```python
from build123d import *

# Parameters (mm, degrees)
F1_DEPTH  = 1525.228
F3_DEPTH  = 1525.228
F5_D      = 19
F5_DEPTH  = 5
F5_TIP    = 5.7081758808
F7_D      = 9
F7_DEPTH  = 5
F7_TIP    = 2.7038727856
F8_R      = 19.05
F9_DEPTH  = 457.2
F10_R     = 7.5
F11_DEPTH = 120
F12_DEPTH = 20
F16_R     = 7.5
F17_DEPTH = 60
F22_R     = 7.5
F23_DEPTH = 60
F28_D     = 15
F28_DEPTH = 5
F28_TIP   = 4.5064546427
F30_D     = 18
F30_DEPTH = 5
F30_TIP   = 5.4077455712
F32_D     = 10
F32_DEPTH = 5
F32_TIP   = 3.0043030951
F33_W     = 75
F33_H     = 1545.228
F34_DEPTH = 2500


# Not quite as in the source:
# - a feature names something its author has since deleted; it is built from what else it names


with BuildPart() as f1:
    # F0 (on Front) → F1 (new body)
    with BuildSketch(Plane.XZ):
        with BuildLine():
            ThreePointArc((0, 12.7), (3.7197438789, 3.7197438789), (12.7, 0))
            Line((12.7, 0), (63.5, 0))
            ThreePointArc((63.5, 0), (72.4802561211, 3.7197438789), (76.2, 12.7))
            Line((76.2, 12.7), (76.2, 63.5))
            ThreePointArc((76.2, 63.5), (72.4802561211, 72.4802561211), (63.5, 76.2))
            Line((63.5, 76.2), (12.7, 76.2))
            ThreePointArc((12.7, 76.2), (3.7197438789, 72.4802561211), (0, 63.5))
            Line((0, 63.5), (0, 12.7))
        make_face()
    extrude(amount=-F1_DEPTH)

    # F2 (on face) → F3 (cut)
    with BuildSketch(Plane.XZ):
        with BuildLine():
            Line((17.4625, 4.7625), (38.1, 4.7625))
            Line((38.1, 4.7625), (58.7375, 4.7625))
            ThreePointArc((58.7375, 4.7625), (67.7177561211, 8.4822438789), (71.4375, 17.4625))
            Line((71.4375, 17.4625), (71.4375, 58.7375))
            ThreePointArc((71.4375, 58.7375), (67.7177561211, 67.7177561211), (58.7375, 71.4375))
            Line((58.7375, 71.4375), (17.4625, 71.4375))
            ThreePointArc((17.4625, 71.4375), (8.4822438789, 67.7177561211), (4.7625, 58.7375))
            Line((4.7625, 58.7375), (4.7625, 17.4625))
            ThreePointArc((4.7625, 17.4625), (8.4822438789, 8.4822438789), (17.4625, 4.7625))
        make_face()
    extrude(amount=-F3_DEPTH, mode=Mode.SUBTRACT)

    # F5
    with Locations(Plane.YZ.offset(76.2)):
        with Locations((1335.228, 46.2), (1105.028, 46.2), (653.528, 46.2), (381.528, 46.2), (179.528, 46.2)):
            Hole(F5_D / 2, depth=F5_DEPTH)
            with Locations((0, 0, -(F5_DEPTH + F5_TIP / 2))):  # 118° drill point
                Cone(0, F5_D / 2, F5_TIP, mode=Mode.SUBTRACT)

    # F7
    with Locations(Plane.YZ.offset(76.2)):
        with Locations((261.933, 31.2), (501.133, 31.2), (760.333, 31.2), (979.533, 31.2), (1218.698, 31.2)):
            Hole(F7_D / 2, depth=F7_DEPTH)
            with Locations((0, 0, -(F7_DEPTH + F7_TIP / 2))):  # 118° drill point
                Cone(0, F7_D / 2, F7_TIP, mode=Mode.SUBTRACT)

    # F8 (on face) → F9 (join)
    with BuildSketch(Plane.XY.offset(76.2)):
        with Locations((38.1, 30)):
            Circle(F8_R)
    extrude(amount=F9_DEPTH)

    # F10 (on face) → F11 (join)
    with BuildSketch(Plane.XY.offset(76.2)):
        with Locations((20.2, 121.55)):
            Circle(F10_R)
    extrude(amount=F11_DEPTH)

    # F12 (add): a face of the model
    f12_faces = [f1.faces().sort_by_distance(p)[0] for p in [
        (1.0776307345, 1525.228, 38.1),
    ]]
    extrude(f12_faces, amount=F12_DEPTH)

    # F16 (on 3pt) → F17 (join)
    with BuildSketch(Plane.XZ.offset(-129.05)):
        with Locations((0, 76.2)):
            Circle(F16_R)
    extrude(amount=-F17_DEPTH)

    # F22 (on 3pt) → F23 (join)
    with BuildSketch(Plane(origin=(0, 1525.228, 0), x_dir=(-1, 0, 0), z_dir=(0, 1, 0))):
        with Locations((0, 76.2)):
            Circle(F22_R)
    extrude(amount=-F23_DEPTH)

    # F28
    with Locations(Plane.YZ.offset(76.2)):
        with Locations((1442.058, 31.2)):
            Hole(F28_D / 2, depth=F28_DEPTH)
            with Locations((0, 0, -(F28_DEPTH + F28_TIP / 2))):  # 118° drill point
                Cone(0, F28_D / 2, F28_TIP, mode=Mode.SUBTRACT)

    # F30
    with Locations(Plane(origin=(0, 0, 0), x_dir=(0, -1, 0), z_dir=(-1, 0, 0))):
        with Locations((-1385.03, 45.756), (-1244.831, 45.756), (-1104.633, 45.756), (-964.435, 45.756), (-263.443, 45.756), (-179.228, 45.756)):
            Hole(F30_D / 2, depth=F30_DEPTH)
            with Locations((0, 0, -(F30_DEPTH + F30_TIP / 2))):  # 118° drill point
                Cone(0, F30_D / 2, F30_TIP, mode=Mode.SUBTRACT)

    # F32
    with Locations(Plane(origin=(0, 0, 0), x_dir=(0, -1, 0), z_dir=(-1, 0, 0))):
        with Locations((-702.728, 47.406), (-350.228, 47.406)):
            Hole(F32_D / 2, depth=F32_DEPTH)
            with Locations((0, 0, -(F32_DEPTH + F32_TIP / 2))):  # 118° drill point
                Cone(0, F32_D / 2, F32_TIP, mode=Mode.SUBTRACT)

    # F33 (on face) → F34 (cut)
    with BuildSketch(Plane(origin=(0, 0, 0), x_dir=(1, 0, 0), z_dir=(0, 0, -1))):
        with Locations((75.6, -772.614)):
            Rectangle(F33_W, F33_H)
    extrude(amount=-F34_DEPTH, mode=Mode.SUBTRACT)


solid = f1.part
```
Geometry: final body of the model. Coordinates: model frame, mm. A direction names the side the tool comes from. Coordinates: 2 decimals unless noted, no trailing zeros. Loops run counter-clockwise (first coordinate to the right, second up) from the corner with the lowest first, then second, coordinate; pieces in that order, holes last. Notation, with made-up numbers: (67.5, 40) -> (121.5, 40) arc R19 ccw to (121.5, 47) -> close; hole circle Ø1 at (-12.75, 46). An arc over 180 degrees is marked (long way). Use a Markdown table: item, result. Add a question column.
(1) Section query C-C, the plane z = 497. Return loops of the section in (x, y).
(2) Section query B-B, the plane z = 151. Return loops of the section in (x, y), plus the area to 3 significant figures.
(3) Section query D-D, the plane y = 1132. Return loops of the section in (x, z), plus the area to 3 significant figures.
(4) Mould query, pull axis Z, two halves, no side actions, for faces 1 (the flat face through (3, 0, 41)), 2 (the flat face through (4.762, 762, 38)), 3 (the flat face through (25, 762, 0)). Classes: pulls with the +Z half, pulls with the -Z half, needs draft (parallel to the pull), parting line crosses it, or undercut.
(5) Access query for faces 4 (the flat face through (3, 1545.228, 41)), 5 (the cylindrical face through (19.055, 30.419, 301.6)). Directions: +Z, -Z, +X, -X, +Y, -Y. A direction counts if a zero-diameter tool reaches every point of the face in a straight line with its end or side. Return the directions, or none.
(6) Pin query (flat end, axial travel): pin 1 Ø8 at (x, z) = (10, 93.5) entering from -Y; pin 2 Ø7.5 at (x, z) = (-0.5, 77.5) entering from -Y; pin 3 Ø23.5 at (y, z) = (179.228, 45.756) entering from -X; pin 4 Ø16.5 at (x, z) = (3, 76.5) entering from +Y. Return the tip coordinate at first contact, or that it passes through.
(7) Section query A-A, the plane y = 30. Return loops of the section in (x, z).
(8) Line query: line 1 along Z through (x, y) = (15, 145); line 2 along Z through (x, y) = (17, 845); line 3 along X through (y, z) = (879, 33). Output: solid intervals per line, ascending.
Answer:
| question | item | result |
|---|---|---|
| 1 | outline | (38.1, 10.95) -> (38.1, 49.05) arc R19.05 ccw to start |
| 2 | outline | circle Ø15 at (20.2, 121.55); (38.1, 10.95) -> (38.1, 49.05) arc R19.05 ccw to start |
| 2 | area | 747 mm^2 |
| 3 | outline | (0, 12.7) arc R12.7 ccw to (12.7, 0) -> (38.1, 0) -> (38.1, 4.76) -> (17.46, 4.76) arc R12.7 cw to (4.76, 17.46) -> (4.76, 58.74) arc R12.7 cw to (17.46, 71.44) -> (38.1, 71.44) -> (38.1, 76.2) -> (12.7, 76.2) arc R12.7 ccw to (0, 63.5) -> close |
| 3 | area | 680 mm^2 |
| 4 | face 1 | needs draft |
| 4 | face 2 | undercut |
| 4 | face 3 | pulls with the -Z half |
| 5 | face 4 | +Z, -Z, +X, -X, +Y |
| 5 | face 5 | +Z, -X |
| 6 | pin 1 | stops at y = 117.33 |
| 6 | pin 2 | stops at y = 129.05 |
| 6 | pin 3 | stops at x = 0 |
| 6 | pin 4 | stops at y = 1545.23 |
| 7 | outline | (0, 12.7) arc R12.7 ccw to (12.7, 0) -> (38.1, 0) -> (38.1, 4.76) -> (17.46, 4.76) arc R12.7 cw to (4.76, 17.46) -> (4.76, 58.74) arc R12.7 cw to (17.46, 71.44) -> (38.1, 71.44) -> (38.1, 533.4) -> (19.05, 533.4) -> (19.05, 76.2) -> (12.7, 76.2) arc R12.7 ccw to (0, 63.5) -> close |
| 8 | line 1 | z = 0 to 5, 71.2 to 76.2 |
| 8 | line 2 | z = 0 to 4.77, 71.43 to 76.2 |
| 8 | line 3 | x = 0 to 4.76 |
